from build123d import *

# Parameters (mm, degrees)
SKETCH_2_R          = 2.750000000000002
SKETCH_2_R_2        = 2.7500000000000018
EXTRUDE_1_DEPTH     = 17.5
SKETCH_8_W          = 23
SKETCH_8_H          = 10.999999999999996
SKETCH_8_W_2        = 17
SKETCH_8_H_2        = 19.999999999999993
CUT_EXTRUDE_2_DEPTH = 56.76961538328914
SKETCH_3_R          = 3.5000000000000004
SKETCH_3_R_2        = 3.500000000000001
CUT_EXTRUDE_1_DEPTH = 6
HOLE_WIZARD_M4_1_D  = 3.3
CUT_EXTRUDE_3_DEPTH = 56.76961538328914
HOLE_WIZARD_M4_2_D  = 3.3
SKETCH_15_W         = 17
SKETCH_15_H         = 5.4999999999999325
CUT_EXTRUDE_5_DEPTH = 5
FILLET_1_R          = 1
FILLET_2_R          = 10


with BuildPart() as part:
    # 草图2 → 凸台-拉伸1 (new, symmetric)
    with BuildSketch(Plane.XY):
        with BuildLine():
            Line((-65, -6.94e-15), (-65, 44.000000000000014))
            Line((-65, 44.000000000000014), (-63.90243902439025, 48.878048780487816))
            ThreePointArc((-63.90243902439025, 48.878048780487816), (-59.99999999999999, 52.00000000000001), (-56.09756097560975, 48.87804878048781))
            Line((-56.09756097560975, 48.87804878048781), (-55.00000000000001, 44.000000000000014))
            Line((-55.00000000000001, 44.000000000000014), (-55.00000000000001, -6.33e-15))
            ThreePointArc((-55.00000000000001, -6.33e-15), (-60, -5.000000000000007), (-65, -6.94e-15))
        make_face()
        with Locations((-60, 38.999999999999986)):
            Circle(SKETCH_2_R, mode=Mode.SUBTRACT)
        with Locations((-60, -6.94e-15)):
            Circle(SKETCH_2_R_2, mode=Mode.SUBTRACT)
    extrude(amount=EXTRUDE_1_DEPTH, both=True)

    # 草图8 → 切除-拉伸2 (cut, through all)
    with BuildSketch(Plane(origin=(-55.00000000000001, 0, 0), x_dir=(0, 0, -1), z_dir=(1, 1.8e-16, 0))):
        with Locations((0, 0.5000000000000178)):
            Rectangle(SKETCH_8_W, SKETCH_8_H)
        with Locations((0, 42.000000000000014)):
            Rectangle(SKETCH_8_W_2, SKETCH_8_H_2)
    extrude(amount=-CUT_EXTRUDE_2_DEPTH, mode=Mode.SUBTRACT)

    # 草图3 → 切除-拉伸1 (cut)
    with BuildSketch(Plane.XY.offset(17.5)):
        with Locations((-60, -6.94e-15)):
            Circle(SKETCH_3_R)
        with Locations(Location((-60, 38.999999999999986, 0), (0, 0, 180))):
            Circle(SKETCH_3_R_2)
    cut_extrude_1 = extrude(amount=-CUT_EXTRUDE_1_DEPTH, mode=Mode.SUBTRACT)

    # M4 螺纹孔1 (through all)
    with Locations(Plane(origin=(-55.00000000000001, 0, 0), x_dir=(0, 0, -1), z_dir=(1, 1.8e-16, 0))):
        with Locations((-12.5, 11.5), (12.5, 11.5), (-12.5, 28), (12.5, 28)):
            Hole(HOLE_WIZARD_M4_1_D / 2)

    # 镜向1: 切除-拉伸1 across plane
    add(cut_extrude_1.mirror(Plane.XY), mode=Mode.SUBTRACT)

    # 草图11 → 切除-拉伸3 (cut, through all)
    with BuildSketch(Plane.ZY.offset(65)):
        with BuildLine():
            Line((-12.5, 23.99999999999997), (-12.5, 15.499999999999966))
            ThreePointArc((-12.5, 15.499999999999966), (-9.67157287525381, 14.328427124746156), (-8.5, 11.499999999999966))
            Line((-8.5, 11.499999999999966), (8.5, 11.499999999999966))
            ThreePointArc((8.5, 11.499999999999966), (9.67157287525381, 14.328427124746156), (12.5, 15.499999999999966))
            Line((12.5, 15.499999999999966), (12.5, 23.99999999999997))
            ThreePointArc((12.5, 23.99999999999997), (9.671572875253812, 25.171572875253784), (8.500000000000004, 27.99999999999997))
            Line((8.500000000000004, 27.99999999999997), (-8.500000000000004, 27.99999999999997))
            ThreePointArc((-8.500000000000004, 27.99999999999997), (-9.671572875253812, 25.171572875253784), (-12.5, 23.99999999999997))
        make_face()
    extrude(amount=-CUT_EXTRUDE_3_DEPTH, mode=Mode.SUBTRACT)

    # M4 螺纹孔2 (through all)
    with Locations(Plane.XY.offset(17.5)):
        with Locations((-60, 19.75), (-60, 48)):
            Hole(HOLE_WIZARD_M4_2_D / 2)

    # 草图15 → 切除-拉伸5 (cut)
    with BuildSketch(Plane.ZY.offset(65)):
        with Locations((0, 8.75)):
            Rectangle(SKETCH_15_W, SKETCH_15_H)
    extrude(amount=-CUT_EXTRUDE_5_DEPTH, mode=Mode.SUBTRACT)

    # 圆角1
    fillet_1_edges = [part.edges().sort_by_distance(p)[0] for p in [
        (-57.5, 11.499999999999968, -8.5),
        (-60, 15.499999999999966, -12.5),
        (-60, 23.99999999999997, -12.5),
        (-60, 27.99999999999997, -8.500000000000002),
        (-60, 27.99999999999997, 8.500000000000002),
        (-60, 23.99999999999997, 12.5),
        (-60, 15.499999999999966, 12.5),
        (-57.5, 11.499999999999968, 8.5),
        (-62.5, 6.000000000000034, -8.5),
        (-62.5, 6.000000000000034, 8.5),
        (-60, 6.000000000000015, -11.5),
        (-60, 6.000000000000015, 11.5),
        (-60.00000000000001, 32.000000000000014, 8.5),
        (-60.00000000000001, 32.000000000000014, -8.5),
    ]]
    fillet(fillet_1_edges, radius=FILLET_1_R)

    # 圆角2
    fillet_2_edges = [part.edges().sort_by_distance(p)[0] for p in [
        (-55.00000000000001, 44.000000000000014, 13),
        (-65, 44.000000000000014, 13),
        (-55.00000000000001, 44.000000000000014, -13),
        (-65, 44.000000000000014, -13),
    ]]
    fillet(fillet_2_edges, radius=FILLET_2_R)


solid = part.part
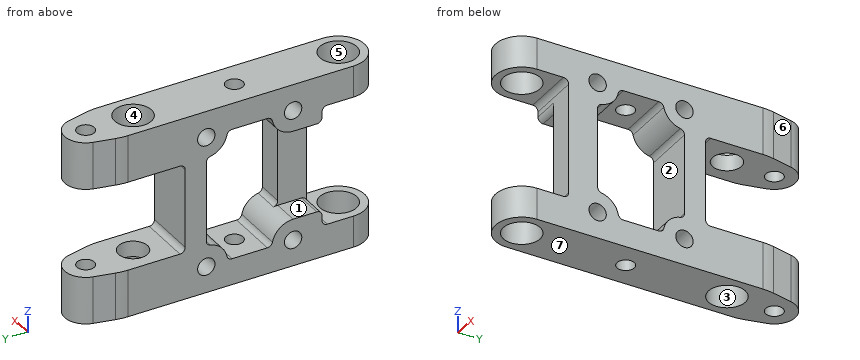
Design review of the part built by this model. Coordinates are the model's own, in mm. Face numbers are marked on the shaded views. A direction names the side the tool comes from. Coordinates: 2 decimals unless noted, no trailing zeros. Loops run counter-clockwise (first coordinate to the right, second up) from the corner with the lowest first, then second, coordinate; pieces in that order, holes last. Notation, with made-up numbers: M 71,-27 L 95,-27 A31 cw 95,10 Z; hole C -7.75,-40 d10. An arc over 180 degrees is marked long. Use one line per item in the form item = value.
(1) For line 1 along Y through (x, z) = (-60, 15.35); line 2 along Y through (x, z) = (-58.75, 6.5); line 3 along Z through (x, y) = (-56.25, 39), list the stretches that pass through material, from the lowest coordinate up. Write a range as from..to.
Return value:
line_1 = -5..-3.5, 3.5..18.1, 21.4..35.5, 42.5..46.35, 49.65..52
line_2 = 6..11.5, 28..32
line_3 = -17.5..-8.5, 8.5..17.5
(2) For the marked faces 1, 2 and 3, list the 3-axis set-ups (+Z, -Z, +X, -X, +Y, -Y) from which the entire face can be reached by the end or side of a thin tool; tool diameter is ignored.
Return value:
face_1 = -X, -Y
face_2 = +X, -X
face_3 = -Z
(3) Consider section B-B (y = 19.75). Write out the cut boundary in (x, z).
Return value:
outline = M -65,-17.5 L -61.65,-17.5 L -61.65,-12.5 L -65,-12.5 Z; M -65,12.5 L -61.65,12.5 L -61.65,17.5 L -65,17.5 Z; M -58.35,-17.5 L -55,-17.5 L -55,-12.5 L -58.35,-12.5 Z; M -58.35,12.5 L -55,12.5 L -55,17.5 L -58.35,17.5 Z
(4) Consider section C-C (z = 15). Write out the cut boundary in (x, y).
Return value:
outline = M -65,0 A5 ccw -55,0 L -55,42.89 A10 ccw -55.24,45.08 L -56.1,48.88 A4 ccw -63.9,48.88 L -64.76,45.08 A10 ccw -65,42.89 Z; hole C -60,0 d7; hole C -60,39 d7; hole C -60,19.75 d3.3; hole C -60,48 d3.3
(5) Consider section A-A (z = -0.5). Write out the cut boundary in (x, y).
Return value:
outline = M -65,28 L -55,28 L -55,32 L -65,32 Z; M -60,6 L -55,6 L -55,11.5 L -60,11.5 Z
(6) Clearance check with flat-ended pins moving along their axes: P1, Ø3, axis at x = -60, y = 1.5, coming from the -Z side; P2, Ø3, axis at x = -58.5, z = 9, coming from the -Y side; P3, Ø3.5, axis at x = -59, y = 38.5, coming from the -Z side. State where each tip first meets the part, or that it passes through.
Return value:
P1 = through
P2 = 6
P3 = -11.5
(7) Draft analysis for pull direction X (two halves, no side actions). For the marked faces 4, 5, 6 and 7, state which applies: pulls with the +X half, pulls with the -X half, needs draft (parallel to the pull), parting line crosses it, or undercut.
Return value:
face_4 = undercut
face_5 = undercut
face_6 = pulls with the +X half
face_7 = needs draft
(8) Consider section D-D (y = 14). Write out the cut boundary in (x, z).
Return value:
outline = M -65,-17.5 L -55,-17.5 L -55,-9.38 L -65,-9.38 Z; M -65,9.38 L -55,9.38 L -55,17.5 L -65,17.5 Z
